from build123d import *

# Parameters (mm, degrees)
ESQUISSE1_W              = 150
ESQUISSE1_H              = 100
BOSS_EXTRU_1_DEPTH       = 5
ENL_V_MAT_EXTRU_1_DEPTH  = 1
ESQUISSE3_R              = 4
ENL_V_MAT_EXTRU_2_DEPTH  = 3
ESQUISSE6_R              = 4
ENL_V_MAT_EXTRU_6_DEPTH  = 3
ESQUISSE7_R              = 4
ENL_V_MAT_EXTRU_8_DEPTH  = 3
ESQUISSE8_R              = 3.982204299
ENL_V_MAT_EXTRU_10_DEPTH = 3


with BuildPart() as part:
    # Esquisse1 → Boss.-Extru.1 (new body)
    with BuildSketch(Plane.XY):
        with Locations((-21.17373101, -10.772659733)):
            Rectangle(ESQUISSE1_W, ESQUISSE1_H)
    extrude(amount=BOSS_EXTRU_1_DEPTH)

    # Esquisse2 → Enlèv. mat.-Extru.1 (cut)
    with BuildSketch(Plane.XY.offset(5)):
        Polygon((-83.17373101, 36.227340267), (39.87366547, 36.227340267), (49.87366547, 26.227340267), (49.87366547, -47.772659733), (39.87366547, -57.772659733), (-83.17373101, -57.772659733), (-93.17373101, -47.772659733), (-93.17373101, 26.227340267), align=None)
    extrude(amount=-ENL_V_MAT_EXTRU_1_DEPTH, mode=Mode.SUBTRACT)

    # Esquisse3 → Enlèv. mat.-Extru.2 (cut)
    with BuildSketch(Plane.XY.offset(5)):
        with Locations((-90.907387201, 34.857641034)):
            Circle(ESQUISSE3_R)
    extrude(amount=-ENL_V_MAT_EXTRU_2_DEPTH, mode=Mode.SUBTRACT)

    # Esquisse6 → Enlèv. mat.-Extru.6 (cut)
    with BuildSketch(Plane.XY.offset(5)):
        with Locations((48.083277729, 34.38144698)):
            Circle(ESQUISSE6_R)
    extrude(amount=-ENL_V_MAT_EXTRU_6_DEPTH, mode=Mode.SUBTRACT)

    # Esquisse7 → Enlèv. mat.-Extru.8 (cut)
    with BuildSketch(Plane.XY.offset(5)):
        with Locations((-91.323021124, -55.986982745)):
            Circle(ESQUISSE7_R)
    extrude(amount=-ENL_V_MAT_EXTRU_8_DEPTH, mode=Mode.SUBTRACT)

    # Esquisse8 → Enlèv. mat.-Extru.10 (cut)
    with BuildSketch(Plane.XY.offset(5)):
        with Locations((48.063086484, -55.947185674)):
            Circle(ESQUISSE8_R)
    extrude(amount=-ENL_V_MAT_EXTRU_10_DEPTH, mode=Mode.SUBTRACT)


solid = part.part
Input: part model. Units: mm. Frame: model coordinates. A direction names the side the tool comes from. Round coordinates to 2 decimals unless told otherwise and drop trailing zeros. Loops run counter-clockwise (first coordinate to the right, second up) from the corner with the lowest first, then second, coordinate; pieces in that order, holes last. Notation, with made-up numbers: M 22,-27.75 L 48,-27.75 A13 cw 48,-17.75 Z; hole C 6.5,24 d9. An arc over 180 degrees is marked long. Answer as CSV lines item,"result". Start each with the question number.
(1) Section A-A, the plane x = -7. Output: boundary loops of the cut face in (y, z).
(2) First-contact query: pin 1 (6.5 mm diameter, centred on x = 48.08, y = 34.38, fed in from -Z); pin 2 (4 mm diameter, centred on x = -91.5, y = 34, fed in from +Z); pin 3 (6 mm diameter, centred on x = -10.5, y = 21.5, fed in from +Z). Flat tips, straight axial feed; report the tip coordinate or a pass-through.
(3) Reachability of faces 4 (the flat face through (-88.2, 31.2, 4.5)), 5 (the flat face through (53.826, -11, 2)) from +Z, -Z, +X, -X, +Y, -Y: full face, straight path, thin tool, end or side. Return the list, or none.
(4) Section B-B, the plane y = 16. Output: boundary loops of the cut face in (x, z).
(5) Line query: line 1 (Y direction, x = -40, z = 4.3); line 2 (Y direction, x = 46.5, z = 2.15); line 3 (X direction, y = -38.5, z = 4.6). Output: solid intervals per line, ascending. Write a range as [from, to].
(6) Draft query along Y for faces 1 (the cylindrical face through (51.9, 35.58, 3.52)), 2 (the flat face through (-22, 39.227, 2)), 3 (the flat face through (-96.174, -11, 2)). Return one class per face: released by +Y, released by -Y, zero draft, split by the parting line, or undercut.
Values found:
1,outline,"M -60.77,0 L 39.23,0 L 39.23,5 L 36.23,5 L 36.23,4 L -57.77,4 L -57.77,5 L -60.77,5 Z"
2,pin 1,"stops at z = 0"
2,pin 2,"stops at z = 2"
2,pin 3,"stops at z = 4"
3,face 4,"+Z"
3,face 5,"+Z, -Z, +X, +Y, -Y"
4,outline,"M -96.17,0 L 53.83,0 L 53.83,5 L 49.87,5 L 49.87,4 L -93.17,4 L -93.17,5 L -96.17,5 Z"
5,line 1,"y = [-60.77, -57.77], [36.23, 39.23]"
5,line 2,"y = [-60.77, -59.61], [-52.28, 30.71], [38.05, 39.23]"
5,line 3,"x = [-96.17, -93.17], [49.87, 53.83]"
6,face 1,"undercut"
6,face 2,"released by +Y"
6,face 3,"zero draft"
